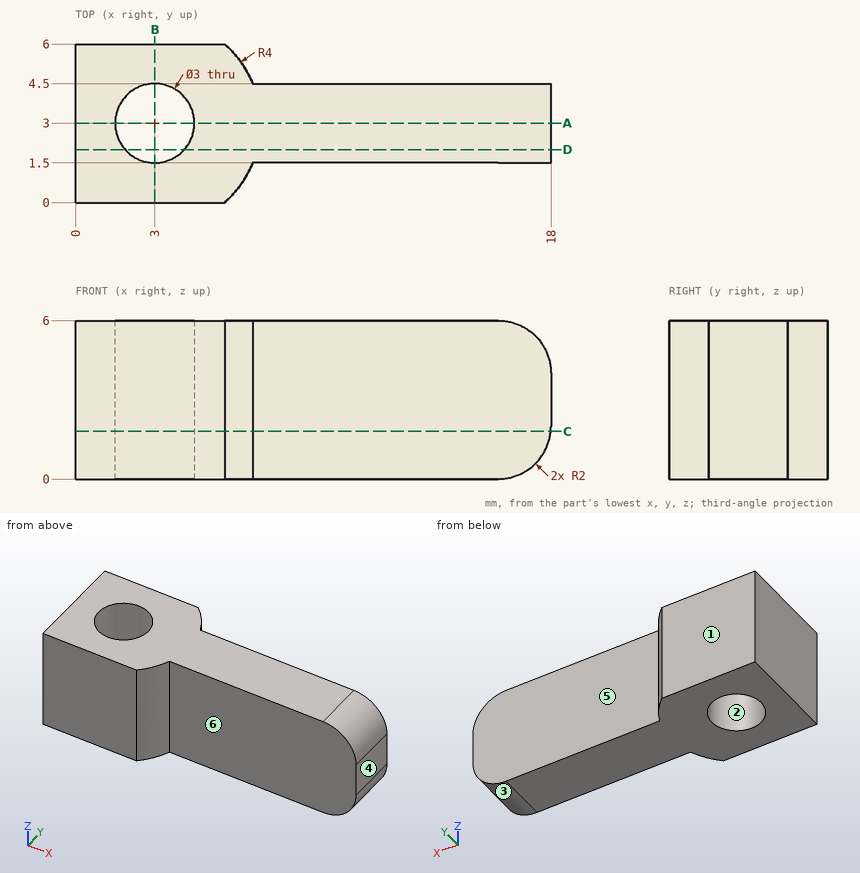
Geometry check sheet. Reference: drawing and pictorial views, mm from the part's lowest x, y, z. A direction names the side the tool comes from. Coordinates: 2 decimals unless noted, no trailing zeros. Loops run counter-clockwise (first coordinate to the right, second up) from the corner with the lowest first, then second, coordinate; pieces in that order, holes last. Notation, with made-up numbers: (-33, 60.25) -> (13, 60.25) arc R21 ccw to (13, 98.25) -> close; hole circle Ø6 at (65, 75.5). An arc over 180 degrees is marked (long way). Put each result on its own line as item: value.
1) Cross-section at D-D on y = 2. Record the boundary of the cut face in (x, z).
Result set:
outline: (0, 0) -> (1.88, 0) -> (1.88, 6) -> (0, 6) -> close; (4.12, 0) -> (16, 0) arc R2 ccw to (18, 2) -> (18, 4) arc R2 ccw to (16, 6) -> (4.12, 6) -> close
2) Tool access check on the marked faces 4, 5 and 6. Record the directions out of +Z, -Z, +X, -X, +Y, -Y that give a thin tool (end or side, any length) a straight path to the whole face; none if there is none.
Result set:
face 4: +Z, -Z, +X, +Y, -Y
face 5: +Z, -Z, +X, +Y
face 6: +Z, -Z, +X, -Y
3) Cross-section at C-C on z = 1.8. Record the boundary of the cut face in (x, y), plus the area to 3 significant figures.
Result set:
outline: (0, 0) -> (5.65, 0) arc R4 ccw to (6.71, 1.5) -> (17.99, 1.5) -> (17.99, 4.5) -> (6.71, 4.5) arc R4 ccw to (5.65, 6) -> (0, 6) -> close; hole circle Ø3 at (3, 3)
area: 65.7 mm^2
4) Cross-section at B-B on x = 3. Record the boundary of the cut face in (y, z), plus the area to 3 significant figures.
Result set:
outline: (0, 0) -> (1.5, 0) -> (1.5, 6) -> (0, 6) -> close; (4.5, 0) -> (6, 0) -> (6, 6) -> (4.5, 6) -> close
area: 18.0 mm^2
5) Release check for a two-part mould opening along Y. For the marked faces 1, 2 and 3 record: released by +Y, released by -Y, zero draft, split by the parting line, or undercut.
Result set:
face 1: released by +Y
face 2: undercut
face 3: zero draft
6) Thickness scan on line 1 (Y direction, x = 3, z = 3.5); line 2 (Y direction, x = 4, z = 2.45); line 3 (X direction, y = 4.25, z = 3.1). Record the ranges inside material, lowest first.
Result set:
line 1: y = 0 to 1.5, 4.5 to 6
line 2: y = 0 to 1.88, 4.12 to 6
line 3: x = 0 to 2.17, 3.83 to 18
7) Cross-section at A-A on y = 3. Record the boundary of the cut face in (x, z), plus the area to 3 significant figures.
Result set:
outline: (0, 0) -> (1.5, 0) -> (1.5, 6) -> (0, 6) -> close; (4.5, 0) -> (16, 0) arc R2 ccw to (18, 2) -> (18, 4) arc R2 ccw to (16, 6) -> (4.5, 6) -> close
area: 88.3 mm^2
8) Gauge pin test, flat ends, axial feed: pin 1 Ø2 at (y, z) = (4.5, 4) entering from -X; pin 2 Ø3 at (x, z) = (12, 4) entering from -Y; pin 3 Ø1.8 at (x, z) = (14, 3) entering from +Y. Record the tip position at first contact, or that the pin passes through.
Result set:
pin 1: stops at x = 0
pin 2: stops at y = 1.5
pin 3: stops at y = 4.5
